For this review, take the finished solid that the model builds, in its own axes (mm). A direction names the side the tool comes from. Coordinates: 2 decimals unless noted, no trailing zeros. Write each loop counter-clockwise with the first axis right and the second up, starting at its lowest first coordinate (ties: lowest second). Pieces come first, ordered by that corner, then holes.
Autodesk Inventor part; units mm, degrees
ref_plane "YZ Plane" through (0, 0, 0) normal (1, 0, 0) x (0, 1, 0)
ref_plane "XZ Plane" through (0, 0, 0) normal (0, 1, 0) x (-1, 0, 0)
ref_plane "XY Plane" through (0, 0, 0) normal (0, 0, 1) x (1, 0, 0)
sketch "Sketch1" plane through (0, 0, 0) normal (1, 0, 0) x (0, 1, 0)
  line L0 (0, 0) -> (58.42, 0) construction
  line L1 (58.42, 0) -> (58.42, -52.705) construction
  line L2 (58.42, -52.705) -> (0, -52.705) construction
  line L3 (0, -52.705) -> (0, 0) construction
  line L4 (0, 0) -> (0, -52.705)
  line L5 (0, -52.705) -> (58.42, -52.705) construction
  line L6 (29.21, -3.81) -> (10.16, -3.81)
  line L7 (10.16, -3.81) -> (10.16, -8.509)
  line L8 (10.16, -8.509) -> (34.29, -8.509)
  line L9 (34.29, -8.509) -> (34.29, -13.589)
  line L10 (34.29, -13.589) -> (15.24, -13.589)
  line L11 (15.24, -13.589) -> (15.24, -18.288)
  line L12 (29.21, -3.81) -> (29.21, 0)
  line L13 (0, 0) -> (29.21, 0) construction
  line L14 (15.24, -18.288) -> (39.37, -18.288)
  line L15 (39.37, -18.288) -> (39.37, -23.368)
  line L16 (39.37, -23.368) -> (20.32, -23.368)
  line L17 (20.32, -23.368) -> (20.32, -28.067)
  line L18 (20.32, -28.067) -> (45.72, -28.067)
  line L19 (45.72, -28.067) -> (45.72, -33.147)
  line L20 (58.42, -52.705) -> (58.42, -47.625)
  line L21 (58.42, -47.625) -> (30.48, -47.625)
  line L22 (30.48, -47.625) -> (30.48, -42.926)
  line L23 (30.48, -42.926) -> (52.07, -42.926)
  line L24 (52.07, -42.926) -> (52.07, -37.846)
  line L25 (52.07, -37.846) -> (25.4, -37.846)
  line L26 (25.4, -37.846) -> (25.4, -33.147)
  line L27 (25.4, -33.147) -> (45.72, -33.147)
  arc A0 (29.21, 0) -> (0, 0) centre (14.605, -61.7976) ccw
  arc A1 (0, -52.705) -> (58.42, -52.705) centre (29.21, 122.6792) ccw
  dimension "d0" = 52.705
  dimension "d1" = 58.42
  dimension "d2" = 4.699
  dimension "d3" = 3.81
  dimension "d5" = 5.08
  dimension "d6" = 5.08
  dimension "d7" = 4.699
  dimension "d8" = 10.16
  dimension "d9" = 19.05
  dimension "d10" = 19.05
  dimension "d11" = 5.08
  dimension "d12" = 4.699
  dimension "d13" = 5.08
  dimension "d14" = 19.05
  dimension "d15" = 5.08
  dimension "d18" = 4.699
  dimension "d19" = 4.699
  dimension "d22" = 5.08
  dimension "d28" = 5.08
  dimension "d35" = 63.5
  dimension "d36" = 177.8
  dimension "d39" = 5.08
  dimension "d40" = 6.35
  dimension "d42" = 5.08
  dimension "d43" = 6.35
  dimension "d44" = 6.35
extrude "Extrusion1" add sketch "Sketch1" against normal blind 4.699
fillet "Fillet1" radius 1.7145 4 edges at (-2.3495, 29.21, 0) (-2.3495, 0, 0) (-2.3495, 0, -52.705) (-2.3495, 58.42, -52.705)
equation "\"d2\" = thick"
equation "\"d6\" = 0.5 * d8"
equation "\"d7\" = thick"
equation "\"d12\" = thick"
equation "\"d13\" = d6"
equation "\"d18\" = thick"
equation "\"d19\" = thick"
equation "\"thick\" = 4.699"
properties part number "Head Frame"
Q1. Add section C-C (y = 32.5). State the section outline as (x, z) points (3 decimals), then the cut area to 3 significant figures.
Ans:
outline: (-4.699, -55.09) - (0, -55.09) - (0, -47.625) - (-4.699, -47.625) - close; (-4.699, -42.926) - (0, -42.926) - (0, -37.846) - (-4.699, -37.846) - close; (-4.699, -33.147) - (0, -33.147) - (0, -28.067) - (-4.699, -28.067) - close; (-4.699, -23.368) - (0, -23.368) - (0, -18.288) - (-4.699, -18.288) - close; (-4.699, -13.589) - (0, -13.589) - (0, -8.509) - (-4.699, -8.509) - close
area: 131 mm2
Q2. Add section A-A (y = 50). State the section outline as (x, z) points (3 decimals), then the cut area to 3 significant figures.
Ans:
outline: (-4.699, -53.901) - (0, -53.901) - (0, -47.625) - (-4.699, -47.625) - close; (-4.699, -42.926) - (0, -42.926) - (0, -37.846) - (-4.699, -37.846) - close
area: 53.4 mm2
Q3. Add section D-D (z = -40). State the section outline as (x, y) points.
Ans:
outline: (-4.7, 0) - (0, 0) - (0, 52.07) - (-4.7, 52.07) - close
Q4. Clearance check with flat-ended pins moving along their axes: pin 1 Ø2.5 at (x, z) = (-2.5, -45) entering from +Y; pin 2 Ø1.5 at (x, z) = (-3, -8.5) entering from +Y; pin 3 Ø1.4 at (x, y) = (-2.5, 21.5) entering from -Z; pin 4 Ø5 at (y, z) = (21, -39.5) entering from +X. State where each tip first meets the part, or that it passes through.
Ans:
pin 1: stops at y = 30.48
pin 2: stops at y = 34.29
pin 3: stops at z = -54.98
pin 4: stops at x = 0
Q5. Tool access review of faces 1 (the flat face through (-4.699, 22, -33)), 2 (the flat face through (-2, 34.29, -11)), 3 (the flat face through (-2, 39, -37.846)): name each direction out of +Z, -Z, +X, -X, +Y, -Y from which nothing blocks a thin tool from reaching the whole face with its end or side.
Ans:
face 1: +Z, -Z, -X, +Y, -Y
face 2: +Z, +X, -X, +Y
face 3: +X, -X, +Y
Q6. For probe 1 along Z at (x, y) = (-1, 31) (3 decimals); probe 2 along Z at (x, y) = (-0.8, 29); probe 3 along Z at (x, y) = (-0.8, 40) (3 decimals), list the stretches that pass through material, from the lowest coordinate up.
Ans:
probe 1: z = -55.112 to -47.625, -42.926 to -37.846, -33.147 to -28.067, -23.368 to -18.288, -13.589 to -8.509
probe 2: z = -55.12 to -37.85, -33.15 to -28.07, -23.37 to -18.29, -13.59 to -8.51, -3.81 to -0.55
probe 3: z = -54.793 to -47.625, -42.926 to -37.846, -33.147 to -28.067
Q7. Draft analysis for pull direction Z (two halves, no side actions). For faces 4 (the flat face through (-2, 20, -3.81)), 5 (the flat face through (-2, 58.42, -49)), 6 (the cylindrical face through (-2.38, 28.82, -0.28)), state which applies: +Z half, -Z half, draft (parallel to the pull), parting line (faces both ways), or undercut.
Ans:
face 4: undercut
face 5: draft
face 6: +Z half
Q8. Add section B-B (x = -1.2). State the section outline as (y, z) points (1 decimal).
Ans:
outline: (0, -51.2) arc R1.7 ccw to (1.4, -52.9) arc R177.8 ccw to (57, -52.9) arc R1.7 ccw to (58.4, -51.2) - (58.4, -47.6) - (30.5, -47.6) - (30.5, -42.9) - (52.1, -42.9) - (52.1, -37.8) - (25.4, -37.8) - (25.4, -33.1) - (45.7, -33.1) - (45.7, -28.1) - (20.3, -28.1) - (20.3, -23.4) - (39.4, -23.4) - (39.4, -18.3) - (15.2, -18.3) - (15.2, -13.6) - (34.3, -13.6) - (34.3, -8.5) - (10.2, -8.5) - (10.2, -3.8) - (29.2, -3.8) - (29.2, -1.4) arc R1.7 ccw to (27.9, 0.3) arc R63.5 ccw to (1.4, 0.3) arc R1.7 ccw to (0, -1.4) - close
